from build123d import *

# Parameters (mm, degrees)
SKETCH_1_R        = 3
EXTRUDE_175_DEPTH = 15
SKETCH_2_R        = 2
EXTRUDE_1_DEPTH   = 15
CHAMFER_1_SIZE    = 0.2
CHAMFER_2_SIZE    = 0.5


with BuildPart() as part:
    # Эскиз1 → Extrude 175 (new body)
    with BuildSketch(Plane.XY):
        Circle(SKETCH_1_R)
    extrude(amount=EXTRUDE_175_DEPTH)

    # Эскиз2 → Бобышка-Вытянуть1 (add)
    with BuildSketch(Plane.XY.offset(15)):
        Circle(SKETCH_2_R)
    extrude(amount=EXTRUDE_1_DEPTH)

    # Фаска1
    chamfer_1_edges = [part.edges().sort_by_distance(p)[0] for p in [
        (-2, 0, 30),
    ]]
    chamfer(chamfer_1_edges, length=CHAMFER_1_SIZE)

    # Фаска2
    chamfer_2_edges = [part.edges().sort_by_distance(p)[0] for p in [
        (-3, 0, 0),
    ]]
    chamfer(chamfer_2_edges, length=CHAMFER_2_SIZE)


solid = part.part
Design review of the part built by this model. Coordinates are the model's own, in mm. A direction names the side the tool comes from. Coordinates: 2 decimals unless noted, no trailing zeros. Order: outer loops, then holes, each group sorted by start corner. A loop starts at its lowest first (then second) coordinate and runs counter-clockwise, first axis right, second up. Notation, with made-up numbers: M 48,65 L 105,65 A16 ccw 105,75 Z; hole C 4,-11.5 d8. An arc over 180 degrees is marked long. Use a Markdown table: item, result.
(1) Wall thickness on probe 1 along X at (y, z) = (-0.05, 20); probe 2 along Z at (x, y) = (-0.5, -2.4); probe 3 along X at (y, z) = (-2.35, 11.25): over which ranges is each line inside the solid? List them lowest first.
Worked answers:
| item | result |
|---|---|
| probe 1 | x = -2 to 2 |
| probe 2 | z = 0 to 15 |
| probe 3 | x = -1.86 to 1.86 |
(2) Add section C-C (z = 16.5). Give the boundary of the cut face in (x, y).
Worked answers:
| item | result |
|---|---|
| outline | C 0,0 d4 |
(3) For P1, Ø3, axis at y = -1.5, z = 22.5, coming from the -X side; P2, Ø2, axis at x = -1, z = 18, coming from the -Y side, all flat-tipped, find the tip position at first contact; note any pin that passes through.
Worked answers:
| item | result |
|---|---|
| P1 | stops at x = -2 |
| P2 | stops at y = -2 |
(4) Add section A-A (x = 0). Give the boundary of the cut face in (y, z).
Worked answers:
| item | result |
|---|---|
| outline | M -3,0.5 L -2.5,0 L 2.5,0 L 3,0.5 L 3,15 L 2,15 L 2,29.8 L 1.8,30 L -1.8,30 L -2,29.8 L -2,15 L -3,15 Z |
(5) For faces 1 (the cylindrical face through (-3, 0, 8)), 2 (the flat face through (1, -2, 15)), list the 3-axis set-ups (+Z, -Z, +X, -X, +Y, -Y) from which the entire face can be reached by the end or side of a thin tool; tool diameter is ignored.
Worked answers:
| item | result |
|---|---|
| face 1 | +Z, -Z |
| face 2 | +Z |
